Source: CAD feature listing. Evaluate the final solid. Frame: model axes, mm. A direction names the side the tool comes from. Coordinates: 2 decimals unless noted, no trailing zeros. Write each loop counter-clockwise with the first axis right and the second up, starting at its lowest first coordinate (ties: lowest second). Pieces come first, ordered by that corner, then holes. Notation, with made-up numbers: M 57.5,43 L 105.5,43 A17 ccw 105.5,75 Z; hole C -30,-19.5 d2. An arc over 180 degrees is marked long. One line per item, written item: value. Start each with the question number.
Item 1: Set-up query: faces 4 (the cylindrical face through (128.289, 0.028, -11.304)), 5 (the cylindrical face through (11.304, 0.028, 128.289)), 6 (the flat face through (-41.24, 0.03, 54.78)), 7 (the flat face through (-23.516, 0.028, -51.312)). Return all of +Z, -Z, +X, -X, +Y, -Y with unobstructed straight access to the full face (end or side cutting, diameter ignored); none if empty.
Item 2: Cut plane D-D, the plane x = 0. Output: boundary loops of the cut face in (y, z), then the cut area to 3 significant figures.
Item 3: Cut plane C-C, the plane y = -0.4. State how many separate pieces and enclosed holes the cut face has, then the cut area to 3 significant figures.
Item 4: Cut plane B-B, the plane x = -97.5. Output: boundary loops of the cut face in (y, z), then the cut area to 3 significant figures.
Item 5: Mould query, pull axis Z, two halves, no side actions, for faces 1 (the flat face through (-2, -2, 18)), 2 (the cylindrical face through (0, 0, -12)), 3 (the cylindrical face through (-61.269, 0.028, -42.694)). Classes: released by +Z, released by -Z, zero draft, split by the parting line, or undercut.
Item 6: Cut plane A-A, the plane z = -62. Output: boundary loops of the cut face in (x, y), then the cut area to 3 significant figures.
Item 7: Ray query, L1, parallel to X at y = 1, z = 16.5; L2, parallel to X at y = -1.35, z = 64.5; L3, parallel to Z at x = -115.5, y = -1.2. Return the intervals inside material, ascending. Write a range as from..to.
Item 8: Pin query (flat end, axial travel): P1, Ø1.2, axis at x = 118.5, y = 1, coming from the -Z side; P2, Ø1.2, axis at x = -111.5, y = 0, coming from the +Z side; P3, Ø1.2, axis at x = 120, y = -1, coming from the +Z side. Return the tip coordinate at first contact, or that it passes through.
```python
from build123d import *

# Parameters (mm, degrees)
SKETCH_1_R          = 1.6
EXTRUDE_1_DEPTH     = 2
SKETCH_2_R          = 1.6
CUT_EXTRUDE_1_DEPTH = 184.891272224
FILLET_1_R          = 10
CUT_EXTRUDE_2_DEPTH = 184.891272224
SKETCH_4_R          = 20
CUT_EXTRUDE_3_DEPTH = 184.891272224
FILLET_3_R          = 20
SKETCH_5_R          = 16
SKETCH_5_R_2        = 18
CUT_EXTRUDE_4_DEPTH = 184.891272224


with BuildPart() as part:
    # 草图1 → 凸台-拉伸1 (new, symmetric)
    with BuildSketch(Plane(origin=(0, 0, 0), x_dir=(1, 0, 0), z_dir=(0, 1, 0))):
        with BuildLine():
            ThreePointArc((-50, 130), (-73.431457505, 73.431457505), (-130, 50))
            Line((-130, 50), (-130, -50))
            ThreePointArc((-130, -50), (-73.431457505, -73.431457505), (-50, -130))
            Line((-50, -130), (50, -130))
            ThreePointArc((50, -130), (73.431457505, -73.431457505), (130, -50))
            Line((130, -50), (130, 50))
            ThreePointArc((130, 50), (73.431457505, 73.431457505), (50, 130))
            Line((50, 130), (-50, 130))
        make_face()
        with Locations(Location((-36, -100.353829072, 0), (0, 0, 270))):
            Circle(SKETCH_1_R, mode=Mode.SUBTRACT)
        with Locations(Location((-72, -38, 0), (0, 0, 270))):
            Circle(SKETCH_1_R, mode=Mode.SUBTRACT)
        with Locations(Location((-5, -52, 0), (0, 0, 270))):
            Circle(SKETCH_1_R, mode=Mode.SUBTRACT)
        with Locations(Location((-5, -4, 0), (0, 0, 270))):
            Circle(SKETCH_1_R, mode=Mode.SUBTRACT)
        with Locations(Location((36, -100.353829072, 0), (0, 0, 270))):
            Circle(SKETCH_1_R, mode=Mode.SUBTRACT)
        with Locations(Location((5, -52, 0), (0, 0, 270))):
            Circle(SKETCH_1_R, mode=Mode.SUBTRACT)
        with Locations(Location((5, -4, 0), (0, 0, 270))):
            Circle(SKETCH_1_R, mode=Mode.SUBTRACT)
        with Locations(Location((72, -38, 0), (0, 0, 270))):
            Circle(SKETCH_1_R, mode=Mode.SUBTRACT)
        with Locations(Location((-36, 24.353829072, 0), (0, 0, 270))):
            Circle(SKETCH_1_R, mode=Mode.SUBTRACT)
        with Locations(Location((36, 24.353829072, 0), (0, 0, 270))):
            Circle(SKETCH_1_R, mode=Mode.SUBTRACT)
    extrude(amount=EXTRUDE_1_DEPTH, both=True)

    # 草图2 → 切除-拉伸1 (cut, through all)
    with BuildSketch(Plane(origin=(0, 2, 0), x_dir=(1, 0, 0), z_dir=(0, 1, 0))):
        with Locations(Location((-52.5, -90, 0), (0, 0, 270))):
            Circle(SKETCH_2_R)
        with Locations(Location((52.5, -90, 0), (0, 0, 90))):
            Circle(SKETCH_2_R)
        with Locations(Location((-90, 52.5, 0), (0, 0, 270))):
            Circle(SKETCH_2_R)
        with Locations(Location((-90, -52.5, 0), (0, 0, 90))):
            Circle(SKETCH_2_R)
        with Locations(Location((90, -52.5, 0), (0, 0, 270))):
            Circle(SKETCH_2_R)
        with Locations(Location((90, 52.5, 0), (0, 0, 90))):
            Circle(SKETCH_2_R)
    extrude(amount=-CUT_EXTRUDE_1_DEPTH, mode=Mode.SUBTRACT)

    # 圆角1
    fillet_1_edges = [part.edges().sort_by_distance(p)[0] for p in [
        (50, 0, 130),
        (-50, 0, 130),
        (-130, 0, 50),
        (-130, 0, -50),
        (-50, 0, -130),
        (50, 0, -130),
        (130, 0, -50),
        (130, 0, 50),
    ]]
    fillet(fillet_1_edges, radius=FILLET_1_R)

    # 草图3 → 切除-拉伸2 (cut, through all)
    with BuildSketch(Plane(origin=(0, 2, 0), x_dir=(1, 0, 0), z_dir=(0, 1, 0))):
        with BuildLine():
            ThreePointArc((-50.4953608, 121.111111111), (-53.997738765, 105.026888717), (-60.717967697, 90))
            Line((-60.717967697, 90), (60.717967697, 90))
            ThreePointArc((60.717967697, 90), (53.997738765, 105.026888717), (50.4953608, 121.111111111))
            ThreePointArc((50.4953608, 121.111111111), (47.223947567, 127.453559925), (40.5572809, 130))
            Line((40.5572809, 130), (-40.5572809, 130))
            ThreePointArc((-40.5572809, 130), (-47.223947567, 127.453559925), (-50.4953608, 121.111111111))
        make_face()
    extrude(amount=-CUT_EXTRUDE_2_DEPTH, mode=Mode.SUBTRACT)

    # 草图4 → 切除-拉伸3 (cut, through all)
    with BuildSketch(Plane(origin=(0, 2, 0), x_dir=(1, 0, 0), z_dir=(0, 1, 0))):
        with BuildLine():
            Line((-30, 90), (-19.724871961, 28.694031744))
            ThreePointArc((-19.724871961, 28.694031744), (-1.658698401, 51.931099308), (20, 32))
            ThreePointArc((20, 32), (19.931099308, 30.341301599), (19.724871961, 28.694031744))
            Line((19.724871961, 28.694031744), (30, 90))
            Line((30, 90), (-30, 90))
        make_face()
        with Locations((0, 32)):
            Circle(SKETCH_4_R)
        with BuildLine():
            ThreePointArc((-25.894156787, -6.299874654), (-23.721640691, -5.891540745), (-22.5, -7.733864491))
            Line((-22.5, -7.733864491), (-22.5, -68.266135509))
            ThreePointArc((-22.5, -68.266135509), (-23.721640691, -70.108459255), (-25.894156787, -69.700125346))
            Line((-25.894156787, -69.700125346), (-57.025039024, -39.433989838))
            ThreePointArc((-57.025039024, -39.433989838), (-57.630882238, -38), (-57.025039024, -36.566010162))
            Line((-57.025039024, -36.566010162), (-25.894156787, -6.299874654))
        make_face()
        with BuildLine():
            ThreePointArc((22.5, -7.733864491), (23.721640691, -5.891540745), (25.894156787, -6.299874654))
            Line((25.894156787, -6.299874654), (57.025039024, -36.566010162))
            ThreePointArc((57.025039024, -36.566010162), (57.630882238, -38), (57.025039024, -39.433989838))
            Line((57.025039024, -39.433989838), (25.894156787, -69.700125346))
            ThreePointArc((25.894156787, -69.700125346), (23.721640691, -70.108459255), (22.5, -68.266135509))
            Line((22.5, -68.266135509), (22.5, -7.733864491))
        make_face()
    extrude(amount=-CUT_EXTRUDE_3_DEPTH, mode=Mode.SUBTRACT)

    # 圆角3
    fillet_3_edges = [part.edges().sort_by_distance(p)[0] for p in [
        (60.717967697, 0, -90),
        (-60.717967697, 0, -90),
        (-30, 0, -90),
        (30, 0, -90),
    ]]
    fillet(fillet_3_edges, radius=FILLET_3_R)

    # 草图5 → 切除-拉伸4 (cut, through all)
    with BuildSketch(Plane(origin=(0, 2, 0), x_dir=(1, 0, 0), z_dir=(0, 1, 0))):
        with BuildLine():
            Line((-37.5, -113), (-18.5, -113))
            ThreePointArc((-18.5, -113), (-17.792893219, -113.292893219), (-17.5, -114))
            Line((-17.5, -114), (-17.5, -122))
            ThreePointArc((-17.5, -122), (-17.792893219, -122.707106781), (-18.5, -123))
            Line((-18.5, -123), (-37.5, -123))
            ThreePointArc((-37.5, -123), (-38.207106781, -122.707106781), (-38.5, -122))
            Line((-38.5, -122), (-38.5, -114))
            ThreePointArc((-38.5, -114), (-38.207106781, -113.292893219), (-37.5, -113))
        make_face()
        with BuildLine():
            Line((-9.5, -108.738101806), (-9.5, -124))
            ThreePointArc((-9.5, -124), (-11.257359313, -128.242640687), (-15.5, -130))
            Line((-15.5, -130), (15.5, -130))
            ThreePointArc((15.5, -130), (11.257359313, -128.242640687), (9.5, -124))
            Line((9.5, -124), (9.5, -108.738101806))
            Line((9.5, -108.738101806), (9.5, -106))
            ThreePointArc((9.5, -106), (0, -109.12560681), (-9.5, -106))
            Line((-9.5, -106), (-9.5, -108.738101806))
        make_face()
        with Locations((0, -93.12560681)):
            Circle(SKETCH_5_R)
        with BuildLine():
            ThreePointArc((17.5, -114), (17.792893219, -113.292893219), (18.5, -113))
            Line((18.5, -113), (37.5, -113))
            ThreePointArc((37.5, -113), (38.207106781, -113.292893219), (38.5, -114))
            Line((38.5, -114), (38.5, -122))
            ThreePointArc((38.5, -122), (38.207106781, -122.707106781), (37.5, -123))
            Line((37.5, -123), (18.5, -123))
            ThreePointArc((18.5, -123), (17.792893219, -122.707106781), (17.5, -122))
            Line((17.5, -122), (17.5, -114))
        make_face()
        with BuildLine():
            ThreePointArc((-11.272727273, -104.480148626), (-9.960882906, -106.431983462), (-9.5, -108.738101806))
            Line((-9.5, -108.738101806), (-9.5, -106))
            ThreePointArc((-9.5, -106), (-10.414126782, -105.272456746), (-11.272727273, -104.480148626))
        make_face()
        with BuildLine():
            ThreePointArc((11.272727273, -104.480148626), (10.414126782, -105.272456746), (9.5, -106))
            Line((9.5, -106), (9.5, -108.738101806))
            ThreePointArc((9.5, -108.738101806), (9.960882906, -106.431983462), (11.272727273, -104.480148626))
        make_face()
        with BuildLine():
            Line((-113, 37.5), (-113, 18.5))
            ThreePointArc((-113, 18.5), (-113.292893219, 17.792893219), (-114, 17.5))
            Line((-114, 17.5), (-122, 17.5))
            ThreePointArc((-122, 17.5), (-122.707106781, 17.792893219), (-123, 18.5))
            Line((-123, 18.5), (-123, 37.5))
            ThreePointArc((-123, 37.5), (-122.707106781, 38.207106781), (-122, 38.5))
            Line((-122, 38.5), (-114, 38.5))
            ThreePointArc((-114, 38.5), (-113.292893219, 38.207106781), (-113, 37.5))
        make_face()
        with BuildLine():
            ThreePointArc((-114, -17.5), (-113.292893219, -17.792893219), (-113, -18.5))
            Line((-113, -18.5), (-113, -37.5))
            ThreePointArc((-113, -37.5), (-113.292893219, -38.207106781), (-114, -38.5))
            Line((-114, -38.5), (-122, -38.5))
            ThreePointArc((-122, -38.5), (-122.707106781, -38.207106781), (-123, -37.5))
            Line((-123, -37.5), (-123, -18.5))
            ThreePointArc((-123, -18.5), (-122.707106781, -17.792893219), (-122, -17.5))
            Line((-122, -17.5), (-114, -17.5))
        make_face()
        with BuildLine():
            ThreePointArc((114, 17.5), (113.292893219, 17.792893219), (113, 18.5))
            Line((113, 18.5), (113, 37.5))
            ThreePointArc((113, 37.5), (113.292893219, 38.207106781), (114, 38.5))
            Line((114, 38.5), (122, 38.5))
            ThreePointArc((122, 38.5), (122.707106781, 38.207106781), (123, 37.5))
            Line((123, 37.5), (123, 18.5))
            ThreePointArc((123, 18.5), (122.707106781, 17.792893219), (122, 17.5))
            Line((122, 17.5), (114, 17.5))
        make_face()
        with BuildLine():
            Line((113, -37.5), (113, -18.5))
            ThreePointArc((113, -18.5), (113.292893219, -17.792893219), (114, -17.5))
            Line((114, -17.5), (122, -17.5))
            ThreePointArc((122, -17.5), (122.707106781, -17.792893219), (123, -18.5))
            Line((123, -18.5), (123, -37.5))
            ThreePointArc((123, -37.5), (122.707106781, -38.207106781), (122, -38.5))
            Line((122, -38.5), (114, -38.5))
            ThreePointArc((114, -38.5), (113.292893219, -38.207106781), (113, -37.5))
        make_face()
        with BuildLine():
            Line((-105.838472485, 9.5), (-124, 9.5))
            ThreePointArc((-124, 9.5), (-128.242640687, 11.257359313), (-130, 15.5))
            Line((-130, 15.5), (-130, -15.5))
            ThreePointArc((-130, -15.5), (-128.242640687, -11.257359313), (-124, -9.5))
            Line((-124, -9.5), (-102.113780207, -9.5))
            ThreePointArc((-102.113780207, -9.5), (-74.727652332, -2.88539126), (-53.379808483, 15.5))
            ThreePointArc((-53.379808483, 15.5), (-74.29932864, 9.138254578), (-85.923486967, 27.657894737))
            ThreePointArc((-85.923486967, 27.657894737), (-92.363349207, 14.720925177), (-105.838472485, 9.5))
        make_face()
        with Locations((-68, 26)):
            Circle(SKETCH_5_R_2)
        with Locations((68, 26)):
            Circle(SKETCH_5_R_2)
        with BuildLine():
            ThreePointArc((130, 15.5), (128.242640687, 11.257359313), (124, 9.5))
            Line((124, 9.5), (105.838472485, 9.5))
            ThreePointArc((105.838472485, 9.5), (92.363349207, 14.720925177), (85.923486967, 27.657894737))
            ThreePointArc((85.923486967, 27.657894737), (85.980861567, 26.829829682), (86, 26))
            ThreePointArc((86, 26), (73.515276634, 8.865773328), (53.379808483, 15.5))
            ThreePointArc((53.379808483, 15.5), (74.727652332, -2.88539126), (102.113780207, -9.5))
            Line((102.113780207, -9.5), (124, -9.5))
            ThreePointArc((124, -9.5), (128.242640687, -11.257359313), (130, -15.5))
            Line((130, -15.5), (130, 15.5))
        make_face()
    extrude(amount=-CUT_EXTRUDE_4_DEPTH, mode=Mode.SUBTRACT)


solid = part.part
```
From the geometry:
1. face 4: +X, +Y, -Y
1. face 5: +Z, +Y, -Y
1. face 6: +Y, -Y
1. face 7: -Z, +Y, -Y
2. outline: M -2,-12 L 2,-12 L 2,77.13 L -2,77.13 Z
2. area: 357 mm²
3. separate pieces: 1
3. enclosed holes: 24
3. area: 29,800 mm²
4. outline: M -2,-56.9 L 2,-56.9 L 2,-11.32 L -2,-11.32 Z; M -2,9.32 L 2,9.32 L 2,56.9 L -2,56.9 Z
4. area: 373 mm²
5. face 1: zero draft
5. face 2: released by -Z
5. face 3: undercut
6. outline: M -87.86,-2 L -25.31,-2 L -25.31,2 L -87.86,2 Z; M 25.31,-2 L 87.86,-2 L 87.86,2 L 25.31,2 Z
6. area: 500 mm²
7. L1: x = -130..-36.39, -22.5..22.5, 36.39..130
7. L2: x = -84.07..-31.24, -22.5..22.5, 31.24..84.07
7. L3: z = -51.33..-38.5, -17.5..-9.5, 9.5..17.5, 38.5..51.33
8. P1: stops at z = -50.92
8. P2: stops at z = 52.31
8. P3: stops at z = 50.71
